Geometry: see drawing. Coordinates: mm, zero at the bounding-box minimum. Coordinates: 2 decimals unless noted, no trailing zeros. Loops run counter-clockwise (first coordinate to the right, second up) from the corner with the lowest first, then second, coordinate; pieces in that order, holes last. Notation, with made-up numbers: (49, 37) -> (99, 37) arc R13 ccw to (99, 45) -> close; hole circle Ø10 at (13, 54). An arc over 180 degrees is marked (long way). Put each result on its own line as item: value. Start each with the question number.
1) Material intervals for L1, parallel to Y at x = 30, z = 6.75; L2, parallel to X at y = 10.5, z = 4; L3, parallel to X at y = 10, z = 3.5 (1 decimal), sorted ascending.
2) Cut plane A-A (y = 7). Return the cut outline in (x, z) (1 decimal).
3) Cut plane B-B (x = 9.5). Return the cut outline in (y, z) (1 decimal), plus the area to 3 significant figures.
4) Contact query for flat-ended pins moving along their axis: P1, Ø3.5, axis at x = 67.59, z = 4.56, coming from the +Y side; P2, Ø1.8, axis at x = 6, y = 7.5, coming from the +Z side (1 decimal). Output: stop coordinate, or through.
5) Cut plane C-C (y = 12). Return the cut outline in (x, z) (1 decimal).
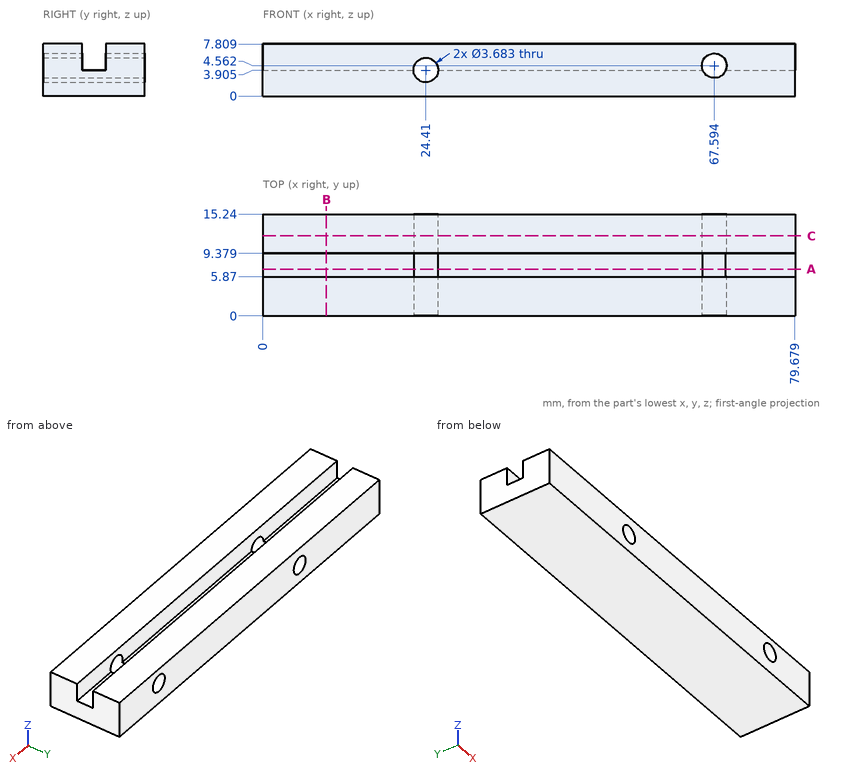
Results found:
1. L1: y = 0 to 5.87, 9.38 to 15.24
1. L2: x = 0 to 22.57, 26.25 to 65.84, 69.35 to 79.68
1. L3: x = 0 to 22.6, 26.2 to 66.1, 69.1 to 79.7
2. outline: (0, 0) -> (79.7, 0) -> (79.7, 3.9) -> (69.3, 3.9) arc R1.8 cw to (65.9, 3.9) -> (26.3, 3.9) arc R1.8 cw to (22.6, 3.9) -> (0, 3.9) -> close
3. outline: (0, 0) -> (15.2, 0) -> (15.2, 7.8) -> (9.4, 7.8) -> (9.4, 3.9) -> (5.9, 3.9) -> (5.9, 7.8) -> (0, 7.8) -> close
3. area: 105 mm2
4. P1: passes through
4. P2: stops at z = 3.9
5. outline: (0, 0) -> (79.7, 0) -> (79.7, 7.8) -> (0, 7.8) -> close; hole circle Ø3.7 at (24.4, 3.9); hole circle Ø3.7 at (67.6, 4.6)
